from build123d import *

# Parameters (mm, degrees)
F2_R     = 15
F3_DEPTH = 40
F4_ANGLE = 90


with BuildPart() as f1:
    # F0 (on Front) → F1 (revolve)
    with BuildSketch(Plane.XZ):
        Polygon((-37.5, 8), (-37.5, 0), (0, 0), (0, 9.672665), (-11, 9.672665), (-11, 12.672665), align=None)
    revolve(axis=Axis((0, 0, -11.012315), (0, 0, 1)))


with BuildPart() as f3:
    # F2 (on Front) → F3 (new body, symmetric)
    with BuildSketch(Plane.XZ):
        with Locations((0, 26)):
            Circle(F2_R)
    extrude(amount=F3_DEPTH, both=True)


with BuildPart() as f4_1:
    # F4: copy of F3
    add(f3.part.rotate(Axis((0, 0, -11.012315), (0, 0, 1)), F4_ANGLE))


with BuildPart() as f1_1:
    add(f1.part)

    # F5: cut F3, F4_1
    add(f3.part, mode=Mode.SUBTRACT)
    add(f4_1.part, mode=Mode.SUBTRACT)


solid = f1_1.part
Design review of the part built by this model. Coordinates are the model's own, in mm. A direction names the side the tool comes from. Give positions to 0.01 mm unless a question says otherwise; leave off trailing zeros. Loops run counter-clockwise (first coordinate to the right, second up) from the corner with the lowest first, then second, coordinate; pieces in that order, holes last. Notation, with made-up numbers: (46.5, 41) - (63.5, 41) arc R29 ccw to (63.5, 67) - close; hole circle Ø9 at (61, 33). An arc over 180 degrees is marked (long way). Use CSV: the item, a comma, the result in double quotes. Start each with the question number.
1. Draft analysis for pull direction X (two halves, no side actions). For faces 3 (the cylindrical face through (4.88, -37.18, 3.94)), 4 (the flat face through (0, 0, 9.673)), 5 (the flat face through (1, -1, 0)), state which applies: released by +X, released by -X, zero draft, split by the parting line, or undercut.
2. Machinability: for faces 1 (the cylindrical face through (-14, 0, 11)), 2 (the cylindrical face through (8.11, -7.43, 10.86)), which of the approach directions +Z, -Z, +X, -X, +Y, -Y give a long, thin tool a straight path to every point of the face, cutting with its end or side? Answer none if there is none.
3. Insertion check: P1, Ø17.5, axis at x = 0, y = 0, coming from the +Z side; P2, Ø5, axis at y = -19, z = 9, coming from the +X side; P3, Ø4, axis at y = 24, z = 3.5, coming from the +X side. Each pin has a flat end and moves straight along its axis. Give the tip position at first contact, or say it passes through.
4. Add section A-A (y = 0). State the section outline as (x, z) points, plus the area to 3 significant figures.
5. Wall thickness on L1, parallel to Y at x = -1, z = 3.5; L2, parallel to Z at x = -11, y = 32.5; L3, parallel to Z at x = -3.5, y = 5: over which ranges is each line inside the solid? List them lowest first.
6. Add section C-C (z = 5.5). State the section outline as (x, y) points.
Results found:
1,face 3,"split by the parting line"
1,face 4,"undercut"
1,face 5,"zero draft"
2,face 1,"+Z, +X, -X"
2,face 2,"+Z"
3,P1,"stops at z = 9.67"
3,P2,"stops at x = 33.57"
3,P3,"stops at x = 30.37"
4,outline,"(-37.5, 0) - (37.5, 0) - (37.5, 8) - (20.49, 11) - (11, 11) - (11, 9.67) - (-11, 9.67) - (-11, 11) - (-20.49, 11) - (-37.5, 8) - close"
4,area,"745 mm²"
5,L1,"y = -37.49 to 37.49"
5,L2,"z = 0 to 8.56"
5,L3,"z = 0 to 9.67"
6,outline,"circle Ø75 at (0, 0)"
